The listing builds one solid part. Answer for the finished solid, in the listing's coordinates (mm). A direction names the side the tool comes from. Round coordinates to 2 decimals unless told otherwise and drop trailing zeros. Loops run counter-clockwise (first coordinate to the right, second up) from the corner with the lowest first, then second, coordinate; pieces in that order, holes last. Notation, with made-up numbers: M 79,41.5 L 104,41.5 A13 cw 104,46.5 Z; hole C 23.5,71.5 d2. An arc over 180 degrees is marked long. Put each result on its own line as item: value. Start each with the question number.
(1) Section B-B, the plane z = 20 is taken. Determine the outline of the cut face in (x, y), then the cut area to 3 significant figures.
(2) Section D-D, the plane x = 252.2 is taken. Determine the outline of the cut face in (y, z).
(3) Straight lines are drawn through the part: line 1 (Z direction, x = 206.2, y = -1.7); line 2 (X direction, y = -4.4, z = 81.5); line 3 (X direction, y = -2, z = 84). For each, find the intervals that lie inside material, in ascending order.
(4) Which of the six approach directions +Z, -Z, +X, -X, +Y, -Y give full straight-line access (tool end or side, diameter ignored) to faces 5 (the face through (134, 0, 64)), 6 (the face through (120, -3, 60))?
(5) A flat-ended cylindrical pin translates along its axis: P1, Ø9, axis at x = 22.2, z = 50, coming from the +Y side. Find the tip coordinate at first contact, or state that the pin passes through.
(6) Section A-A, the plane x = 81 is taken. Determine the outline of the cut face in (y, z).
(7) Determine the mould class of faces 1 (the face through (0, -3, 66)), 2 (the face through (200.7, -3, 25.1)), 3 (the face through (138, -3, 130)), 4 (the face through (134, -3, 0)) for opening direction Z: released by +Z, released by -Z, zero draft, split by the parting line, or undercut.
(8) Section C-C, the plane y = -5.1 is taken. Count the separate pieces of the cut face and the enclosed holes in it, then the cut area to 3 significant figures.
Autodesk Fusion 360 part; units mm, degrees
sketch "Sketch1" plane through (0, 0, 0) normal (0, 1, 0) x (1, 0, 0)
  line L0 (0, 0) -> (272.2, 0)
  line L1 (272.2, 0) -> (272.2, -130)
  line L2 (272.2, -130) -> (0, -130)
  line L3 (0, -130) -> (0, 0)
  dimension "d1" = 272.2
  dimension "d2" = 130
extrude "Extrude1" add sketch "Sketch1" against normal blind 6
sketch "Sketch2" plane through (0, -6, 0) normal (0, -1, 0) x (1, 0, 0)
  line L0 (272.2, 130) -> (0, 130)
  line L1 (0, 130) -> (0, 0)
  line L2 (0, 0) -> (272.2, 0)
  line L3 (272.2, 0) -> (272.2, 130)
  line L4 (70, 40) -> (100, 40)
  arc A0 (100, 40) -> (100, 80) centre (100, 60) ccw
  line L5 (100, 80) -> (70, 80)
  arc A1 (70, 80) -> (70, 40) centre (70, 60) ccw
  line L6 (50, 60) -> (120, 60) construction
  circle A2 centre (252.2, 110) radius 7.5
  circle A3 centre (206.2, 110) radius 7.5
  circle A4 centre (160.2, 110) radius 7.5
  circle A5 centre (114.2, 110) radius 7.5
  circle A6 centre (68.2, 110) radius 7.5
  circle A7 centre (252.2, 80) radius 7.5
  circle A8 centre (206.2, 80) radius 7.5
  circle A9 centre (252.2, 50) radius 7.5
  circle A10 centre (206.2, 50) radius 7.5
  circle A11 centre (160.2, 50) radius 7.5
  circle A12 centre (22.2, 110) radius 7.5
  circle A13 centre (22.2, 80) radius 7.5
  circle A14 centre (22.2, 50) radius 7.5
  circle A15 centre (252.2, 20) radius 7.5
  circle A16 centre (206.2, 20) radius 7.5
  circle A17 centre (160.2, 20) radius 7.5
  circle A18 centre (114.2, 20) radius 7.5
  circle A19 centre (68.2, 20) radius 7.5
  circle A20 centre (22.2, 20) radius 7.5
  circle A21 centre (160.2, 80) radius 7.5
  dimension "d5" = 40
  dimension "d6" = 50
  dimension "d8" = 40
  dimension "d9" = 15
  dimension "d10" = 20
  dimension "d11" = 20
  dimension "d14" = -230
  dimension "d15" = -90
extrude "Extrude2" cut sketch "Sketch2" against normal up to surface (6 mm away) contours L4 A0 L5 A1 | A2 | A3 | A4 | A5 | A6 | A7 | A8 | A9 | A10 | A11 | A12 | A13 | A14 | A15 | A16 | A17 | A18 | A19 | A20 | A21
Recorded:
1. outline: M 0,-6 L 14.7,-6 L 14.7,0 L 0,0 Z; M 29.7,-6 L 60.7,-6 L 60.7,0 L 29.7,0 Z; M 75.7,-6 L 106.7,-6 L 106.7,0 L 75.7,0 Z; M 121.7,-6 L 152.7,-6 L 152.7,0 L 121.7,0 Z; M 167.7,-6 L 198.7,-6 L 198.7,0 L 167.7,0 Z; M 213.7,-6 L 244.7,-6 L 244.7,0 L 213.7,0 Z; M 259.7,-6 L 272.2,-6 L 272.2,0 L 259.7,0 Z
1. area: 1,090 mm²
2. outline: M -6,0 L 0,0 L 0,12.5 L -6,12.5 Z; M -6,27.5 L 0,27.5 L 0,42.5 L -6,42.5 Z; M -6,57.5 L 0,57.5 L 0,72.5 L -6,72.5 Z; M -6,87.5 L 0,87.5 L 0,102.5 L -6,102.5 Z; M -6,117.5 L 0,117.5 L 0,130 L -6,130 Z
3. line 1: z = 0 to 12.5, 27.5 to 42.5, 57.5 to 72.5, 87.5 to 102.5, 117.5 to 130
3. line 2: x = 0 to 14.85, 29.55 to 152.85, 167.55 to 198.85, 213.55 to 244.85, 259.55 to 272.2
3. line 3: x = 0 to 15.86, 28.54 to 153.86, 166.54 to 199.86, 212.54 to 245.86, 258.54 to 272.2
4. face 5: +Z, -Z, +X, -X, +Y
4. face 6: +Y, -Y
5. P1: passes through
6. outline: M -6,0 L 0,0 L 0,40 L -6,40 Z; M -6,80 L 0,80 L 0,130 L -6,130 Z
7. face 1: zero draft
7. face 2: undercut
7. face 3: released by +Z
7. face 4: released by -Z
8. separate pieces: 1
8. enclosed holes: 21
8. area: 29,400 mm²
